```python
from build123d import *

# Parameters (mm, degrees)
SWEEP_THIN1_PROFILE_R   = 7.5
SWEEP_THIN1_PROFILE_R_2 = 5
CUT_EXTRUDE2_DEPTH      = 208.777034922
CUT_EXTRUDE2_DEPTH_BACK = 208.777034922
SKETCH34_R              = 9


with BuildPart() as part:
    # Sweep-Thin1: sweep along a path in Sketch1
    with BuildLine(Plane(origin=(0, 0, 0), x_dir=(1, 0, 0), z_dir=(0, 1, 0))) as sweep_thin1_path:
        Line((0, 90), (140.362285796, 47.891314261))
        ThreePointArc((140.362285796, 47.891314261), (175.994891518, 0), (140.362285796, -47.891314261))
        Line((140.362285796, -47.891314261), (0, -90))
    # Sweep-Thin1 profile (on start of the path) → Sweep-Thin1 (sweep)
    with BuildSketch(Plane(origin=(0, 0, -90), x_dir=(-0.2873478855663455, 0, 0.9578262852211514), z_dir=(0.9578262852211514, 0, 0.2873478855663455))):
        Circle(SWEEP_THIN1_PROFILE_R)
        Circle(SWEEP_THIN1_PROFILE_R_2, mode=Mode.SUBTRACT)
    sweep(path=sweep_thin1_path.line)

    # Sketch34 → Cut-Extrude2 (cut, two sides: drawn at the far end of the back side and taken through both)
    with BuildSketch(Plane.XY.offset(-CUT_EXTRUDE2_DEPTH_BACK)):
        Circle(SKETCH34_R)
    extrude(amount=CUT_EXTRUDE2_DEPTH + CUT_EXTRUDE2_DEPTH_BACK, mode=Mode.SUBTRACT)


solid = part.part
```
Part model, mm, in its own coordinate system. Round coordinates to 2 decimals unless told otherwise and drop trailing zeros. Write each loop counter-clockwise with the first axis right and the second up, starting at its lowest first coordinate (ties: lowest second). Pieces come first, ordered by that corner, then holes. Notation, with made-up numbers: (88, 28) -> (110, 28) arc R15 cw to (110, 48) -> close; hole circle Ø10 at (26, -5). An arc over 180 degrees is marked (long way). Return JSON: item names as keys, results as strings. Group by question number.
Q1. Saw through at B-B on x = 40.5. State how many separate pieces and enclosed holes the cut face has, plus the area to 3 significant figures.
Q2. Probe L1, parallel to Z at x = 120.5, y = 3.25; L2, parallel to Z at x = 95, y = -3; L3, parallel to X at y = -0.5, z = -19. List the from-to ranges inside material, lowest first. Write a range as [from, to].
Q3. Saw through at A-A on y = -2.75. Write the cut outline in (x, z), plus the area to 3 significant figures.
Q4. Pin check, flat tips, straight feed: pin 1 (10 mm diameter, centred on x = 38.5, z = -69, fed in from +Y); pin 2 (5 mm diameter, centred on x = 82.5, y = -2.5, fed in from -Z); pin 3 (8 mm diameter, centred on x = 82.5, y = -4, fed in from +Z). Stop position of each tip, or through.
Answer:
{
 "1": {"separate pieces": "2", "enclosed holes": "2", "area": "205 mm2"},
 "2": {"L1": "[-60.91, -57.82], [-49.88, -46.79], [46.79, 49.88], [57.82, 60.91]", "L2": "[-68.68, -65.68], [-57.32, -54.32], [54.32, 57.32], [65.68, 68.68]", "L3": "[164.03, 166.81], [177.58, 180.25]"},
 "3": {"outline": "(8.57, -94.71) -> (142.37, -54.57) arc R56.98 ccw to (142.37, 54.57) -> (8.57, 94.71) -> (8.57, 91.79) -> (141.56, 51.89) arc R54.18 cw to (141.56, -51.89) -> (8.57, -91.79) -> close; (8.57, -83.07) -> (139.16, -43.89) arc R45.82 ccw to (139.16, 43.89) -> (8.57, 83.07) -> (8.57, 80.14) -> (138.36, 41.21) arc R43.02 cw to (138.36, -41.21) -> (8.57, -80.14) -> close", "area": "2,260 mm2"},
 "4": {"pin 1": "y = 6.31", "pin 2": "z = -73.62", "pin 3": "z = 73.86"}
}
